Build history of the part. All positions in model axes, mm. A direction names the side the tool comes from. Coordinates: 2 decimals unless noted, no trailing zeros. Order: outer loops, then holes, each group sorted by start corner. A loop starts at its lowest first (then second) coordinate and runs counter-clockwise, first axis right, second up. Notation, with made-up numbers: M 83,84.5 L 123,84.5 A24 cw 123,115.5 Z; hole C 13,26.5 d11. An arc over 180 degrees is marked long. Write item = value, one per line. Start each with the question number.
Q1. Band-saw the part on B-B on x = 0. Write the cut outline in (y, z), plus the area to 4 significant figures.
Q2. Band-saw the part on A-A on y = 0. Write the cut outline in (x, z).
Q3. Drill centre lines: probe 1 along X at (y, z) = (-0.2, 24.5); probe 2 along X at (y, z) = (-1.5, 42.5); probe 3 along Y at (x, z) = (-0.65, 11). Where is each one in solid material? Low to high.
Q4. Pin check, flat tips, straight feed: P1, Ø0.6, axis at x = 0, y = -0.5, coming from the +Z side; P2, Ø1.5, axis at y = 1.5, z = 47.5, coming from the -X side; P3, Ø3, axis at x = 2, z = 15, coming from the +Y side. Stop position of each tip, or through.
Q5. Band-saw the part on C-C on z = 25. Write the cut outline in (x, y), plus the area to 3 significant figures.
Q6. 3-axis set-ups, long thin cutter, end or side, ignore diameter. For faces 4 (the face through (2, 0, 49)), 5 (the face through (0, -1, 54)), 6 (the face through (-1.1, -0.4, 59)): which of +Z, -Z, +X, -X, +Y, -Y reach the whole face in a straight line?
Q7. Pull direction Y, two halves, no side cores. Call faces 1 (the face through (-2.5, 0.1, 29.1)), 2 (the face through (0, 0, 49)), 3 (the face through (0, 0, 0)): released by +Y, released by -Y, zero draft, split by the parting line, or undercut.
```python
from build123d import *

# Parameters (mm, degrees)
SKETCH1_R           = 2.5
BOSS_EXTRUDE1_DEPTH = 59
SKETCH2_R           = 1
CUT_EXTRUDE1_DEPTH  = 10
CHAMFER1_SIZE       = 0.5
SKETCH3_W           = 1.530069222
SKETCH3_H           = 4.686409644
CUT_EXTRUDE2_DEPTH  = 10


with BuildPart() as part:
    # Sketch1 → Boss-Extrude1 (new body)
    with BuildSketch(Plane.XY):
        Circle(SKETCH1_R)
    extrude(amount=BOSS_EXTRUDE1_DEPTH)

    # Sketch2 → Cut-Extrude1 (cut)
    with BuildSketch(Plane.XY.offset(59)):
        Circle(SKETCH2_R)
    extrude(amount=-CUT_EXTRUDE1_DEPTH, mode=Mode.SUBTRACT)

    # Chamfer1
    chamfer1_edges = [part.edges().sort_by_distance(p)[0] for p in [
        (-2.5, 0, 0),
        (-2.5, 0, 59),
    ]]
    chamfer(chamfer1_edges, length=CHAMFER1_SIZE)

    # Sketch3 → Cut-Extrude2 (cut)
    with BuildSketch(Plane.XY.offset(59)):
        with Locations((2.265034611, -0.329447038)):
            Rectangle(SKETCH3_W, SKETCH3_H)
    extrude(amount=-CUT_EXTRUDE2_DEPTH, mode=Mode.SUBTRACT)


solid = part.part
```
Recorded:
q1.outline = M -2.5,0.5 L -2,0 L 2,0 L 2.5,0.5 L 2.5,58.5 L 2,59 L 1,59 L 1,49 L -1,49 L -1,59 L -2,59 L -2.5,58.5 Z
q1.area = 274.5 mm2
q2.outline = M -2.5,0.5 L -2,0 L 2,0 L 2.5,0.5 L 2.5,49 L 1.5,49 L 1.5,59 L 1,59 L 1,49 L -1,49 L -1,59 L -2,59 L -2.5,58.5 Z
q3.probe_1 = -2.49 to 2.49
q3.probe_2 = -2 to 2
q3.probe_3 = -2.41 to 2.41
q4.P1 = 49
q4.P2 = -2.38
q4.P3 = 2.45
q5.outline = C 0,0 d5
q5.area = 19.6 mm2
q6.face_4 = +Z, +X, +Y, -Y
q6.face_5 = +Z
q6.face_6 = +Z, +X, -X, +Y, -Y
q7.face_1 = split by the parting line
q7.face_2 = undercut
q7.face_3 = zero draft
